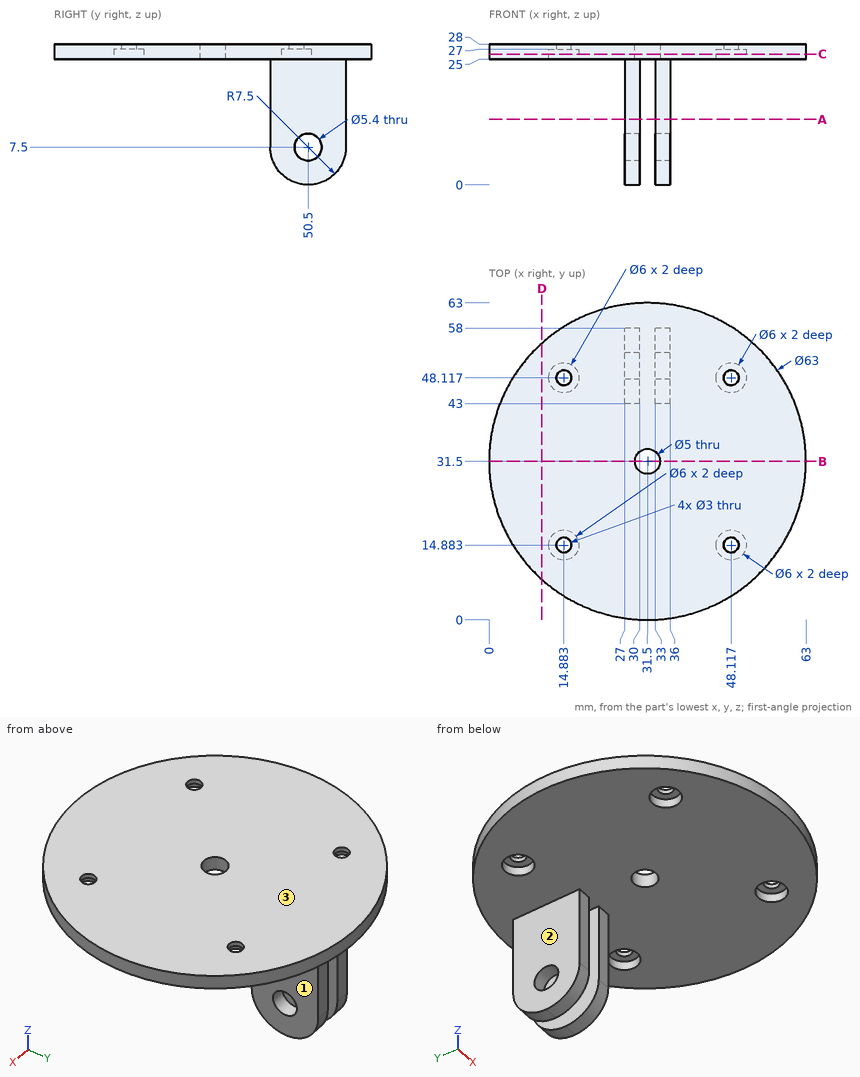
Part print with two shaded views. Sizes in mm from the minimum x, y, z corner. A direction names the side the tool comes from. Coordinates: 2 decimals unless noted, no trailing zeros. Order: outer loops, then holes, each group sorted by start corner. A loop starts at its lowest first (then second) coordinate and runs counter-clockwise, first axis right, second up.
(1) Saw through at B-B, the plane y = 31.5. Write the cut outline in (x, z).
Solution:
outline: (0, 25) - (29, 25) - (29, 28) - (0, 28) - close; (34, 25) - (63, 25) - (63, 28) - (34, 28) - close
(2) Which spindle directions (+Z, -Z, +X, -X, +Y, -Y) get a long thin tool onto all of the face, cutting with end or side? Do the marked faces 1, 2 and 3. Say none if no direction does.
Solution:
face 1: -Z, +X, +Y, -Y
face 2: -Z, -X, +Y, -Y
face 3: +Z, +X, -X, +Y, -Y
(3) Saw through at A-A, the plane z = 13. Write the cut outline in (x, y).
Solution:
outline: (27, 43) - (30, 43) - (30, 58) - (27, 58) - close; (33, 43) - (36, 43) - (36, 58) - (33, 58) - close
(4) Saw through at C-C, the plane z = 26. Write the cut outline in (x, y).
Solution:
outline: circle Ø63 at (31.5, 31.5); hole circle Ø6 at (14.88, 14.88); hole circle Ø6 at (14.88, 48.12); hole circle Ø5 at (31.5, 31.5); hole circle Ø6 at (48.12, 14.88); hole circle Ø6 at (48.12, 48.12)
(5) Pin check, flat tips, straight feed: pin 1 Ø4.5 at (y, z) = (53.5, 16.5) entering from -X; pin 2 Ø6.5 at (x, y) = (48, 48) entering from -Z; pin 3 Ø5 at (x, z) = (9.5, 22) entering from -Y; pin 4 Ø0.9 at (x, z) = (34.5, 12.5) entering from +Y. Stop position of each tip, or through.
Solution:
pin 1: stops at x = 27
pin 2: stops at z = 25
pin 3: passes through
pin 4: stops at y = 58
(6) Drill centre lines: L1, parallel to X at y = 15, z = 26; L2, parallel to Z at x = 33.65, y = 50.5; L3, parallel to Y at x = 34, z = 16.75. Where is each one in solid material? Low to high.
Solution:
L1: x = 4.67 to 11.89, 17.88 to 45.12, 51.11 to 58.33
L2: z = 0 to 4.8, 10.2 to 28
L3: y = 43 to 58
(7) Saw through at D-D, the plane x = 10.5. Write the cut outline in (y, z), and give its area (3 significant figures).
Solution:
outline: (8.02, 25) - (54.98, 25) - (54.98, 28) - (8.02, 28) - close
area: 141 mm2
